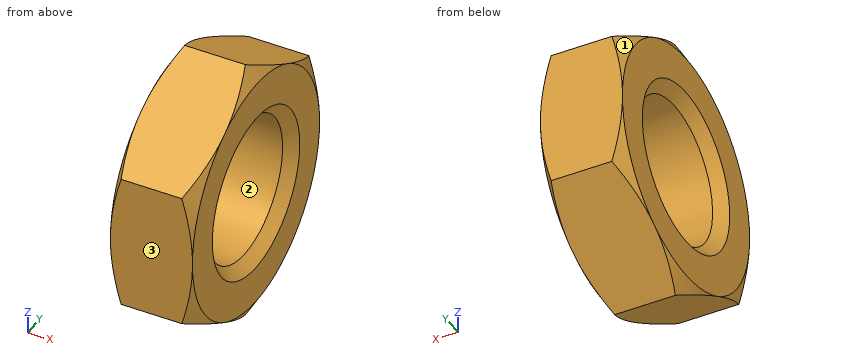
```python
from build123d import *

# Parameters (mm, degrees)
SKETCH1_R      = 9.5
EXTRUDE1_DEPTH = 5.5
SMUSSO1_SIZE   = 1.5


# Read off the part's stored shape, not the designer's step: Cut-Extrude1
with BuildPart() as part:
    # Sketch1 → Extrude1 (new, symmetric)
    with BuildSketch(Plane(origin=(0, 0, 0), x_dir=(0, 0, -1), z_dir=(1, 0, 0))):
        Polygon((18.475208614, 0), (9.237604307, 16), (-9.237604307, 16), (-18.475208614, 0), (-9.237604307, -16), (9.237604307, -16), align=None)
        Circle(SKETCH1_R, mode=Mode.SUBTRACT)
    extrude(amount=EXTRUDE1_DEPTH, both=True)

    # Cut-Extrude1 outline → Cut-Extrude1 (revolve, cut)
    with BuildSketch(Plane.YX):
        Polygon((18.475208616, 5.500000004), (15.999999996, 5.500000004), (18.475208616, 4.070937639), align=None)
    cut_extrude1 = revolve(axis=Axis((0, 0, 0), (1, 0, 0)), mode=Mode.SUBTRACT)

    # Mirror1: Cut-Extrude1 across plane
    add(cut_extrude1.mirror(Plane(origin=(0, 0, 0), x_dir=(0, 0, 1), z_dir=(1, 0, 0))), mode=Mode.SUBTRACT)

    # Smusso1
    smusso1_edges = [part.edges().sort_by_distance(p)[0] for p in [
        (-5.5, 0, 9.5),
        (5.5, 0, 9.5),
    ]]
    chamfer(smusso1_edges, length=SMUSSO1_SIZE)


solid = part.part
```
Here's how the part is built. I have some questions about the finished solid (model axes, mm). Face numbers are marked on the shaded views. Give positions to 0.01 mm unless a question says otherwise; leave off trailing zeros. Order: outer loops, then holes, each group sorted by start corner. A loop starts at its lowest first (then second) coordinate and runs counter-clockwise, first axis right, second up. Notation, with made-up numbers: (-26, 60.5) -> (-6, 60.5) arc R20 cw to (-6, 94.5) -> close; hole circle Ø11 at (-31.75, 75.5). An arc over 180 degrees is marked (long way). Use CSV: the item, a comma, the result in double quotes. Start each with the question number.
Item 1: Suppose I cut it at A-A (x = -1.5). List the corners of the cut face in (y, z) for me.
Item 2: I'm going to push flat-ended pins straight in: P1, Ø12, axis at y = 6.5, z = 1, coming from the -X side; P2, Ø4, axis at x = 3.5, y = 6, coming from the +Z side; P3, Ø2, axis at x = 2, y = 2, coming from the -Z side; P4, Ø1, axis at x = -1.5, y = -7, coming from the -Z side. Where does each tip first touch, or does it pass through?
Item 3: Thinking about a two-plate mould opening in Z: for the marked faces 1, 2 and 3, which applies, pulls with the +Z half, pulls with the -Z half, needs draft (parallel to the pull), parting line crosses it, or undercut?
Item 4: If I drill on probe 1 along Z at (x, y) = (3.25, 7.5); probe 2 along Z at (x, y) = (3.75, 8.5); probe 3 along Y at (x, z) = (1.5, 3), over which ranges is the centre line in solid material (lowest first)? Write a range as [from, to].
Answer block:
1,outline,"(-16, -9.24) -> (0, -18.48) -> (16, -9.24) -> (16, 9.24) -> (0, 18.48) -> (-16, 9.24) -> close; hole circle Ø19 at (0, 0)"
2,P1,"stops at x = -5.5"
2,P2,"stops at z = 16.17"
2,P3,"stops at z = -17.9"
2,P4,"stops at z = -14.72"
3,face 1,"pulls with the +Z half"
3,face 2,"undercut"
3,face 3,"needs draft"
4,probe 1,"z = [-14.15, -5.83], [5.83, 14.15]"
4,probe 2,"z = [-13.57, -4.24], [4.24, 13.57]"
4,probe 3,"y = [-16, -9.01], [9.01, 16]"
